Design review of the part built by this model. Coordinates are the model's own, in mm. A direction names the side the tool comes from. Give positions to 0.01 mm unless a question says otherwise; leave off trailing zeros. Write each loop counter-clockwise with the first axis right and the second up, starting at its lowest first coordinate (ties: lowest second). Pieces come first, ordered by that corner, then holes.
```python
from build123d import *

# Parameters (mm, degrees)
SALIENTE_EXTRUIR1_DEPTH = 37
CORTAR_EXTRUIR1_DEPTH   = 10


with BuildPart() as part:
    # Croquis1 → Saliente-Extruir1 (new body)
    with BuildSketch(Plane.XY):
        Polygon((55.350000047, 77.336068513), (100.017938292, 0), (104.347630379, 2.500753173), (59.766286021, 79.886836776), (54.412620908, 89.152214546), (50.000000028, 86.602540366), align=None)
    extrude(amount=SALIENTE_EXTRUIR1_DEPTH)

    # Croquis2 → Cortar-Extruir1 (cut)
    with BuildSketch(Plane(origin=(79.427815776, 45.757565725, 0), x_dir=(0, 0, -1), z_dir=(0.866497897, 0.499180723, 0))):
        Polygon((-33.424409531, 19.532383801), (-33.424409531, -19.467616199), (-28.124409531, -19.467616199), (-28.124409531, -0.028001757), (-28.124409531, 0.092769359), (-28.124409531, 19.532383801), align=None)
    extrude(amount=-CORTAR_EXTRUIR1_DEPTH, mode=Mode.SUBTRACT)


solid = part.part
```
(1) Mouldability with a two-part tool opening along Z and no side actions: class faces 3 (the face through (102.15, 1.23, 18.24)), 4 (the face through (77, 45, 37)), 5 (the face through (67.508, 61.433, 30.737)) as pulls with the +Z half, pulls with the -Z half, needs draft (parallel to the pull), parting line crosses it, or undercut.
Resolved:
face 3: needs draft
face 4: pulls with the +Z half
face 5: undercut
(2) Consider section B-B, the plane x = 71. Give the boundary of the cut face in (y, z).
Resolved:
outline: (50.24, 0) - (60.39, 0) - (60.39, 28.12) - (50.24, 28.12) - close; (50.24, 33.42) - (60.39, 33.42) - (60.39, 37) - (50.24, 37) - close
(3) Consider section C-C, the plane z = 9. Give the boundary of the cut face in (x, y).
Resolved:
outline: (50, 86.6) - (55.35, 77.34) - (100.02, 0) - (104.35, 2.5) - (59.77, 79.89) - (54.41, 89.15) - close
(4) Tool access review of faces 1 (the face through (77, 45, 0)), 2 (the face through (86.995, 27.65, 30.812)): name each direction out of +Z, -Z, +X, -X, +Y, -Y from which nothing blocks a thin tool from reaching the whole face with its end or side.
Resolved:
face 1: -Z, +X, -X, +Y, -Y
face 2: -X, +Y
(5) Consider section D-D, the plane y = 28. Give the boundary of the cut face in (x, z), then the cut area to 3 significant figures.
Resolved:
outline: (83.85, 0) - (89.66, 0) - (89.66, 37) - (83.85, 37) - (83.85, 33.42) - (87.6, 33.42) - (87.6, 28.12) - (83.85, 28.12) - close
area: 195 mm2
(6) Clearance check with flat-ended pins moving along their axes: P1, Ø12, axis at y = 14.5, z = 9, coming from the -X side; P2, Ø5, axis at y = 25.5, z = 19, coming from the -X side; P3, Ø12, axis at y = 19.5, z = 10.5, coming from the -X side. State where each tip first meets the part, or that it passes through.
Resolved:
P1: stops at x = 88.18
P2: stops at x = 83.85
P3: stops at x = 85.29
(7) Consider section A-A, the plane y = 46.5. Give the boundary of the cut face in (x, z).
Resolved:
outline: (73.16, 0) - (79, 0) - (79, 28.12) - (73.16, 28.12) - close; (73.16, 33.42) - (79, 33.42) - (79, 37) - (73.16, 37) - close
(8) To check wall thickness, follow L1, parallel to X at y = 85.5, z = 28; L2, parallel to X at y = 20, z = 27.5; L3, parallel to Y at x = 53, z = 10. State the ranges of each line that lie inside material, in increasing order.
Resolved:
L1: x = 50.64 to 56.52
L2: x = 88.47 to 94.27
L3: y = 81.41 to 88.34
